Design review of the part built by this model. Coordinates are the model's own, in mm. A direction names the side the tool comes from. Round coordinates to 2 decimals unless told otherwise and drop trailing zeros. Write each loop counter-clockwise with the first axis right and the second up, starting at its lowest first coordinate (ties: lowest second). Pieces come first, ordered by that corner, then holes. Notation, with made-up numbers: (49.25, -19.5) - (79.25, -19.5) arc R32 cw to (79.25, 6.5) - close; hole circle Ø8 at (-29.5, 42.5). An arc over 180 degrees is marked (long way). Use one line per item in the form item = value.
```python
from build123d import *

# Parameters (mm, degrees)
F0_W     = 234.762548
F0_H     = 46.762416
F0_W_2   = 230.000048
F0_H_2   = 41.999916
F1_DEPTH = 3.175
F2_W     = 234.762548
F2_H     = 46.762416
F3_DEPTH = 2.38125
F5_DEPTH = 5.55625
F6_R     = 2.15265
F7_DEPTH = 5.55625
F8_R     = 0.79375
F9_DEPTH = 3.175


# Not quite as in the source:
# - a length typed as a fraction of an inch, garbled in the dataset ("3 / 203.2 mm" for 3/8 in), is restored


with BuildPart() as f1:
    # F0 (on Top) → F1 (new body)
    with BuildSketch(Plane.XY):
        Rectangle(F0_W, F0_H)
        Rectangle(F0_W_2, F0_H_2, mode=Mode.SUBTRACT)
    extrude(amount=F1_DEPTH)

    # F2 (on face) → F3 (join)
    with BuildSketch(Plane(origin=(0, 0, 0), x_dir=(1, 0, 0), z_dir=(0, 0, -1))):
        Rectangle(F2_W, F2_H)
    extrude(amount=F3_DEPTH)

    # F4 (on face) → F5 (join, through all)
    with BuildSketch(Plane(origin=(0, 0, -2.38125), x_dir=(1, 0, 0), z_dir=(0, 0, -1))):
        with BuildLine():
            Line((-121.408854552, -20.241406366), (-117.381274, -23.381208))
            Line((-117.381274, -23.381208), (-117.381274, -9.9112329577))
            Line((-117.381274, -9.9112329577), (-121.7751040378, -14.3050629955))
            ThreePointArc((-121.7751040378, -14.3050629955), (-122.9299921425, -17.3557849119), (-121.408854552, -20.241406366))
        make_face()
        with BuildLine():
            Line((-117.381274, 9.9112329577), (-117.381274, 23.381208))
            Line((-117.381274, 23.381208), (-121.408854552, 20.241406366))
            ThreePointArc((-121.408854552, 20.241406366), (-122.9299921425, 17.3557849119), (-121.7751040378, 14.3050629955))
            Line((-121.7751040378, 14.3050629955), (-117.381274, 9.9112329577))
        make_face()
        with BuildLine():
            Line((117.381274, -9.9112329577), (117.381274, -23.381208))
            Line((117.381274, -23.381208), (121.408854552, -20.241406366))
            ThreePointArc((121.408854552, -20.241406366), (122.9299921425, -17.3557849119), (121.7751040378, -14.3050629955))
            Line((121.7751040378, -14.3050629955), (117.381274, -9.9112329577))
        make_face()
        with BuildLine():
            Line((121.408854552, 20.241406366), (117.381274, 23.381208))
            Line((117.381274, 23.381208), (117.381274, 9.9112329577))
            Line((117.381274, 9.9112329577), (121.7751040378, 14.3050629955))
            ThreePointArc((121.7751040378, 14.3050629955), (122.9299921425, 17.3557849119), (121.408854552, 20.241406366))
        make_face()
    extrude(amount=-F5_DEPTH)

    # F6 (on face) → F7 (cut, through all)
    with BuildSketch(Plane(origin=(0, 0, -2.38125), x_dir=(1, 0, 0), z_dir=(0, 0, -1))):
        with Locations((-118.968774, -17.1113930333)):
            Circle(F6_R)
        with Locations((-118.968774, 17.1113930333)):
            Circle(F6_R)
        with Locations((118.968774, 17.1113930333)):
            Circle(F6_R)
        with Locations((118.968774, -17.1113930333)):
            Circle(F6_R)
    extrude(amount=-F7_DEPTH, mode=Mode.SUBTRACT)

    # F8 (on face) → F9 (cut, through all)
    with BuildSketch(Plane.XY.offset(3.175)):
        with Locations((-115.000024, 20.999958)):
            Circle(F8_R)
        with Locations((-115.000024, -20.999958)):
            Circle(F8_R)
        with Locations((115.000024, -20.999958)):
            Circle(F8_R)
        with Locations((115.000024, 20.999958)):
            Circle(F8_R)
    extrude(amount=-F9_DEPTH, mode=Mode.SUBTRACT)


solid = f1.part
```
Q1. Machinability: for faces 1 (the cylindrical face through (-120.677, -15.802, 0.358)), 2 (the flat face through (-119.55, 12.08, 0.36)), 3 (the flat face through (119.55, -12.08, 0.36)), 4 (the flat face through (119.37, 21.83, 0.36)), 5 (the flat face through (-2, 0, 0)), which of the approach directions +Z, -Z, +X, -X, +Y, -Y give a long, thin tool a straight path to every point of the face, cutting with its end or side? Answer none if there is none.
Calculated:
face_1 = +Z, -Z
face_2 = +Z, -Z, -X
face_3 = +Z, -Z, +X
face_4 = +Z, -Z, +X, +Y
face_5 = +Z
Q2. To check wall thickness, follow line 1 along X through (y, z) = (-17.5, 1.45); line 2 along Y through (x, z) = (-8, 0.1); line 3 along X through (y, z) = (-4, 0.45). State the ranges of each line that lie inside material, in increasing order. Write a range as from..to.
Calculated:
line_1 = -122.92..-121.09, -116.85..-115, 115..116.85, 121.09..122.92
line_2 = -23.38..-21, 21..23.38
line_3 = -117.38..-115, 115..117.38
Q3. We need section C-C on z = 2.2. Write out the cut boundary in (x, y), then the cut area to 3 significant figures.
Calculated:
outline = (-121.78, -14.31) arc R3.97 ccw to (-121.41, -20.24) - (-117.38, -23.38) - (117.38, -23.38) - (121.41, -20.24) arc R3.97 ccw to (121.78, -14.31) - (117.38, -9.91) - (117.38, 9.91) - (121.78, 14.31) arc R3.97 ccw to (121.41, 20.24) - (117.38, 23.38) - (-117.38, 23.38) - (-121.41, 20.24) arc R3.97 ccw to (-121.78, 14.31) - (-117.38, 9.91) - (-117.38, -9.91) - close; hole circle Ø4.31 at (-118.97, -17.11); hole circle Ø4.31 at (-118.97, 17.11); hole (-115, -20.21) arc R0.79 ccw (long way) to (-114.21, -21) - (114.21, -21) arc R0.79 ccw (long way) to (115, -20.21) - (115, 20.21) arc R0.79 ccw (long way) to (114.21, 21) - (-114.21, 21) arc R0.79 ccw (long way) to (-115, 20.21) - close; hole circle Ø4.31 at (118.97, -17.11); hole circle Ø4.31 at (118.97, 17.11)
area = 1,440 mm2
Q4. We need section B-B on y = -7.5. Write out the cut boundary in (x, z) (3 decimals).
Calculated:
outline = (-117.381, -2.381) - (117.381, -2.381) - (117.381, 3.175) - (115, 3.175) - (115, 0) - (-115, 0) - (-115, 3.175) - (-117.381, 3.175) - close
Q5. We need section A-A on x = -39. Write out the cut boundary in (y, z) (3 decimals).
Calculated:
outline = (-23.381, -2.381) - (23.381, -2.381) - (23.381, 3.175) - (21, 3.175) - (21, 0) - (-21, 0) - (-21, 3.175) - (-23.381, 3.175) - close
Q6. Draft analysis for pull direction Y (two halves, no side actions). For faces 6 (the flat face through (-119.37, -21.83, 0.36)), 7 (the flat face through (-2, 0, -2.381)), 8 (the cylindrical face through (122.927, 17.403, 0.358)), state which applies: released by +Y, released by -Y, zero draft, split by the parting line, or undercut.
Calculated:
face_6 = released by -Y
face_7 = zero draft
face_8 = undercut
Q7. For P1, Ø1, axis at y = 10, z = 1, coming from the +X side; P2, Ø22, axis at x = 46, y = -3, coming from the +Z side; P3, Ø4, axis at x = -118.97, y = 17.11, coming from the -Z side; P4, Ø1.7, axis at y = -4.5, z = 0, coming from the +X side, all flat-tipped, find the tip position at first contact; note any pin that passes through.
Calculated:
P1 = 117.97
P2 = 0
P3 = through
P4 = 117.38
